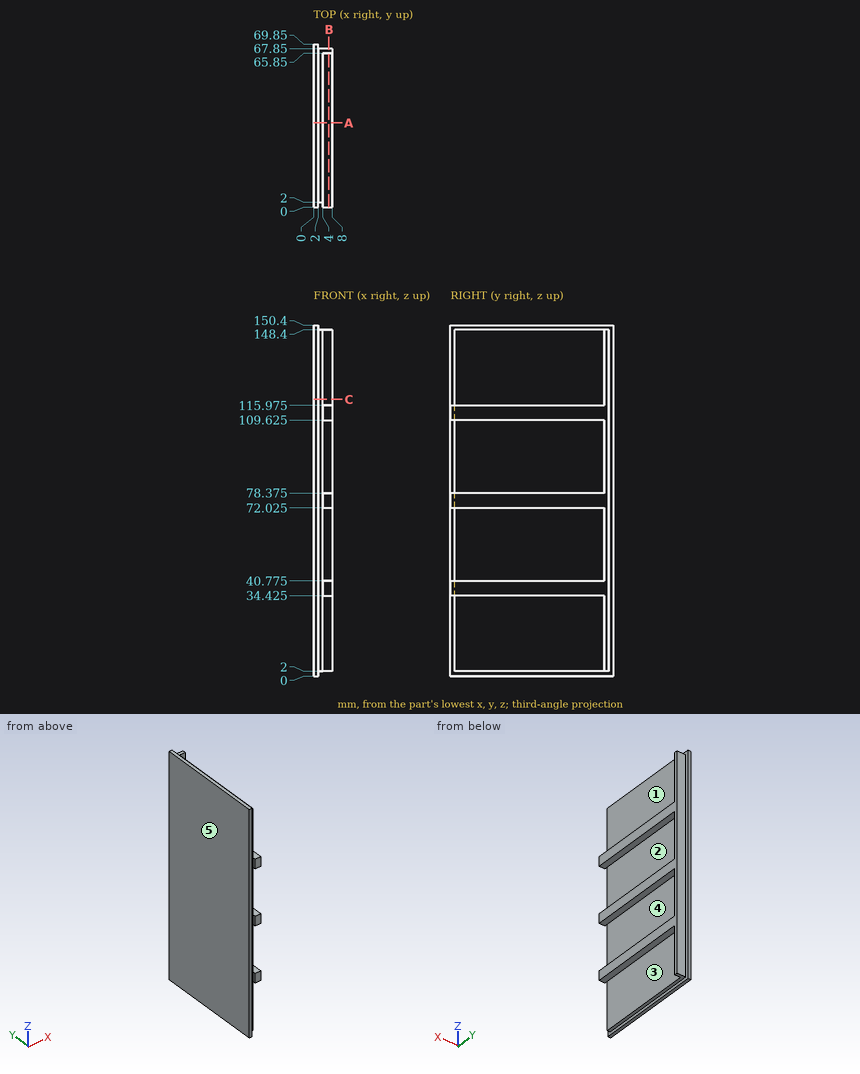
Geometry: see drawing. Coordinates: mm, zero at the bounding-box minimum. A direction names the side the tool comes from. Round coordinates to 2 decimals unless told otherwise and drop trailing zeros. Loops run counter-clockwise (first coordinate to the right, second up) from the corner with the lowest first, then second, coordinate; pieces in that order, holes last. Notation, with made-up numbers: (8, 36) - (45, 36) arc R9 ccw to (45, 51) - close; hole circle Ø5 at (74, 17.5). An arc over 180 degrees is marked (long way). Use CSV: the item, a comma, the result in double quotes.
Q1. Section query C-C, the plane z = 118.5. Output: boundary loops of the cut face in (x, y).
Reported:
outline,"(0, 0) - (2, 0) - (2, 2) - (4, 2) - (4, 65.85) - (8, 65.85) - (8, 67.85) - (2, 67.85) - (2, 69.85) - (0, 69.85) - close"
Q2. Reachability of the marked faces 1, 2 and 3 from +Z, -Z, +X, -X, +Y, -Y: full face, straight path, thin tool, end or side. Return the list, or none.
Reported:
face 1,"+Z, +X, -Y"
face 2,"+X, -Y"
face 3,"-Z, +X, -Y"
Q3. Section query B-B, the plane x = 6.5. Output: boundary loops of the cut face in (y, z) (3 decimals).
Reported:
outline,"(0, 34.425) - (65.85, 34.425) - (65.85, 2) - (67.85, 2) - (67.85, 148.4) - (65.85, 148.4) - (65.85, 115.975) - (0, 115.975) - (0, 109.625) - (65.85, 109.625) - (65.85, 78.375) - (0, 78.375) - (0, 72.025) - (65.85, 72.025) - (65.85, 40.775) - (0, 40.775) - close"
Q4. Mould query, pull axis Z, two halves, no side actions, for the marked faces 4 and 5. Classes: pulls with the +Z half, pulls with the -Z half, needs draft (parallel to the pull), parting line crosses it, or undercut.
Reported:
face 4,"undercut"
face 5,"needs draft"
Q5. Pin query (flat end, axial travel): pin 1 Ø3 at (x, z) = (6.5, 128) entering from -Y; pin 2 Ø1.5 at (x, y) = (6, 26) entering from -Z (3 decimals); pin 3 Ø2 at (y, z) = (58.5, 127) entering from +X. Return the tip coordinate at first contact, or that it passes through.
Reported:
pin 1,"y = 65.85"
pin 2,"z = 34.425"
pin 3,"x = 4"
Q6. Section query A-A, the plane y = 36. Output: boundary loops of the cut face in (x, z) (3 decimals), then the cut area to 3 significant figures.
Reported:
outline,"(0, 0) - (2, 0) - (2, 2) - (4, 2) - (4, 34.425) - (8, 34.425) - (8, 40.775) - (4, 40.775) - (4, 72.025) - (8, 72.025) - (8, 78.375) - (4, 78.375) - (4, 109.625) - (8, 109.625) - (8, 115.975) - (4, 115.975) - (4, 148.4) - (2, 148.4) - (2, 150.4) - (0, 150.4) - close"
area,"670 mm^2"
Q7. Ray query, line 1 along Z through (x, y) = (6.5, 62) (3 decimals); line 2 along Z through (x, y) = (3.25, 11); line 3 along X through (y, z) = (62, 17). Return the intervals inside material, ascending.
Reported:
line 1,"34.425 to 40.775, 72.025 to 78.375, 109.625 to 115.975"
line 2,"2 to 148.4"
line 3,"0 to 4"
